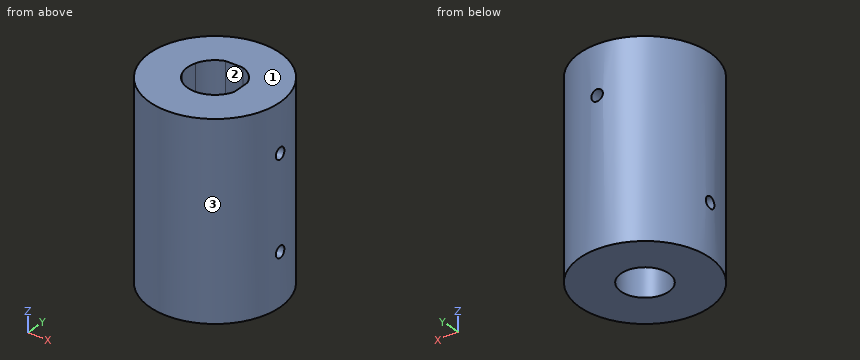
from build123d import *

# Parameters (mm, degrees)
F0_R      = 17
F0_R_2    = 6.25
F1_DEPTH  = 50
F3_DEPTH  = 25
F4_DEPTH  = 25
F5_R      = 1.5
F6_DEPTH  = 25
F7_R      = 1.5
F8_DEPTH  = 25
F9_R      = 1.5
F10_DEPTH = 50


with BuildPart() as f1:
    # F0 (on Top) → F1 (new body)
    with BuildSketch(Plane.XY):
        Circle(F0_R)
        Circle(F0_R_2, mode=Mode.SUBTRACT)
        Circle(F0_R_2)
    extrude(amount=F1_DEPTH)

    # F0 (on Top) → F3 (cut)
    with BuildSketch(Plane.XY):
        Circle(F0_R_2)
    extrude(amount=F3_DEPTH, mode=Mode.SUBTRACT)

    # F2 (on face) → F4 (cut)
    with BuildSketch(Plane.XY.offset(50)):
        with BuildLine():
            Line((6.75, -2.2810359489), (6.75, 2.2810359489))
            ThreePointArc((6.75, 2.2810359489), (5.038135816, 5.038135816), (2.2810359489, 6.75))
            Line((2.2810359489, 6.75), (-2.2810359489, 6.75))
            ThreePointArc((-2.2810359489, 6.75), (-5.038135816, 5.038135816), (-6.75, 2.2810359489))
            Line((-6.75, 2.2810359489), (-6.75, -2.2810359489))
            ThreePointArc((-6.75, -2.2810359489), (-5.038135816, -5.038135816), (-2.2810359489, -6.75))
            Line((-2.2810359489, -6.75), (2.2810359489, -6.75))
            ThreePointArc((2.2810359489, -6.75), (5.038135816, -5.038135816), (6.75, -2.2810359489))
        make_face()
        with BuildLine():
            Line((-6.75, -2.2810359489), (-6.75, 2.2810359489))
            ThreePointArc((-6.75, 2.2810359489), (-7.125, 0), (-6.75, -2.2810359489))
        make_face()
        with BuildLine():
            ThreePointArc((-2.2810359489, -6.75), (0, -7.125), (2.2810359489, -6.75))
            Line((2.2810359489, -6.75), (-2.2810359489, -6.75))
        make_face()
    extrude(amount=-F4_DEPTH, mode=Mode.SUBTRACT)

    # F5 (on face) → F6 (cut)
    with BuildSketch(Plane(origin=(6.75, 0, 0), x_dir=(0, -1, 0), z_dir=(-1, 0, 0))):
        with Locations((0, 37.5)):
            Circle(F5_R)
    extrude(amount=-F6_DEPTH, mode=Mode.SUBTRACT)

    # F7 (on face) → F8 (cut)
    with BuildSketch(Plane.XZ.offset(-6.75)):
        with Locations((0, 37.5)):
            Circle(F7_R)
    extrude(amount=-F8_DEPTH, mode=Mode.SUBTRACT)

    # F9 (on Right) → F10 (cut, symmetric)
    with BuildSketch(Plane.YZ):
        with Locations((0, 13.5)):
            Circle(F9_R)
    extrude(amount=F10_DEPTH, both=True, mode=Mode.SUBTRACT)


solid = f1.part
Design review of the part built by this model. Coordinates are the model's own, in mm. Face numbers are marked on the shaded views. Give positions to 0.01 mm unless a question says otherwise; leave off trailing zeros. Write each loop counter-clockwise with the first axis right and the second up, starting at its lowest first coordinate (ties: lowest second). Pieces come first, ordered by that corner, then holes. Notation, with made-up numbers: M 84,10.25 L 94,10.25 A27 ccw 94,30.25 Z; hole C 10,77.25 d1. An arc over 180 degrees is marked long. Answer as a JSON object with one key per item and string values. Group by question number.
1) We need section D-D (z = 17). Give the boundary of the cut face in (x, y).
2) Mouldability with a two-part tool opening along Y and no side actions: class the marked faces 1, 2 and 3 as released by +Y, released by -Y, zero draft, split by the parting line, or undercut.
3) Clearance check with flat-ended pins moving along their axes: pin 1 Ø5 at (y, z) = (12, 7.5) entering from -X; pin 2 Ø2.5 at (y, z) = (0, 13.5) entering from -X; pin 3 Ø6 at (x, z) = (-11, 33.5) entering from -Y; pin 4 Ø1.5 at (y, z) = (4.5, 5.5) entering from -X. State where each tip first meets the part, or that it passes through.
4) For line 1 along X through (y, z) = (0, 8.25); line 2 along Z through (x, y) = (0, 11), list the stretches that pass through material, from the lowest coordinate up.
5) We need section B-B (y = 0). Give the boundary of the cut face in (x, z) (3 decimals).
6) We need section A-A (x = 0). Give the boundary of the cut face in (y, z) (3 decimals), and give its area (3 significant figures).
7) We need section C-C (z = 37.5). Give the boundary of the cut face in (x, y) (3 decimals), and give its area (3 significant figures).
Answer key:
{
 "1": {"outline": "C 0,0 d34; hole C 0,0 d12.5"},
 "2": {"face 1": "zero draft", "face 2": "undercut", "face 3": "split by the parting line"},
 "3": {"pin 1": "stops at x = -14.1", "pin 2": "passes through", "pin 3": "stops at y = -15", "pin 4": "stops at x = -16.58"},
 "4": {"line 1": "x = -17 to -6.25, 6.25 to 17", "line 2": "z = 0 to 36, 39 to 50"},
 "5": {"outline": "M -17,0 L -6.25,0 L -6.25,12 L -17,12 Z; M -17,15 L -6.25,15 L -6.25,25 L -7.125,25 L -7.125,50 L -17,50 Z; M 6.25,0 L 17,0 L 17,12 L 6.25,12 Z; M 6.25,15 L 17,15 L 17,36 L 6.75,36 L 6.75,25 L 6.25,25 Z; M 6.75,39 L 17,39 L 17,50 L 6.75,50 Z"},
 "6": {"outline": "M -17,0 L -6.25,0 L -6.25,25 L -7.125,25 L -7.125,50 L -17,50 Z; M 6.25,0 L 17,0 L 17,36 L 6.75,36 L 6.75,25 L 6.25,25 Z; M 6.75,39 L 17,39 L 17,50 L 6.75,50 Z", "area": "1,010 mm²"},
 "7": {"outline": "M -2.281,6.75 L -1.5,6.75 L -1.5,16.934 A17 ccw long 16.934,-1.5 L 6.75,-1.5 L 6.75,-2.281 A7.125 cw long Z; M 1.5,6.75 L 2.281,6.75 A7.125 cw 6.75,2.281 L 6.75,1.5 L 16.934,1.5 A17 ccw 1.5,16.934 Z", "area": "689 mm²"}
}
